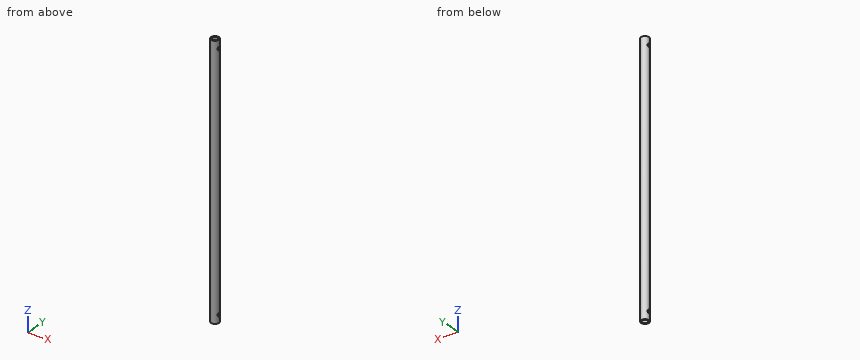
from build123d import *

# Parameters (mm, degrees)
ESQUISSE1_R                  = 3
ESQUISSE1_R_2                = 2
BOSS_EXTRU_1_DEPTH           = 199
ENL_V_MAT_EXTRU_1_DEPTH      = 200.045220993
ENL_V_MAT_EXTRU_1_DEPTH_BACK = 200.045220993
ESQUISSE2_R                  = 1.25


with BuildPart() as part:
    # Esquisse1 → Boss.-Extru.1 (new body)
    with BuildSketch(Plane.XY):
        Circle(ESQUISSE1_R)
        Circle(ESQUISSE1_R_2, mode=Mode.SUBTRACT)
    extrude(amount=BOSS_EXTRU_1_DEPTH)

    # Esquisse2 → Enlèv. mat.-Extru.1 (cut, two sides: drawn at the far end of the back side and taken through both)
    with BuildSketch(Plane(origin=(0, 0, 0), x_dir=(0, 0, -1), z_dir=(1, 0, 0)).offset(-ENL_V_MAT_EXTRU_1_DEPTH_BACK)):
        with Locations((-6, 0)):
            Circle(ESQUISSE2_R)
        with Locations((-193, 0)):
            Circle(ESQUISSE2_R)
    extrude(amount=ENL_V_MAT_EXTRU_1_DEPTH + ENL_V_MAT_EXTRU_1_DEPTH_BACK, mode=Mode.SUBTRACT)


solid = part.part
Input: part model. Units: mm. Frame: model coordinates. Give positions to 0.01 mm unless a question says otherwise; leave off trailing zeros. Loops run counter-clockwise (first coordinate to the right, second up) from the corner with the lowest first, then second, coordinate; pieces in that order, holes last. Notation, with made-up numbers: (32, 4.5) -> (76, 4.5) arc R19 ccw to (76, 36.5) -> close; hole circle Ø6 at (42.5, 17.5). An arc over 180 degrees is marked (long way). Answer as a JSON object with one key per item and string values. Group by question number.
Item 1: Cut plane A-A, the plane x = 0. Return the cut outline in (y, z).
Item 2: Pin query (flat end, axial travel): P1, Ø1, axis at x = -1, z = 147.5, coming from the +Y side; P2, Ø1.5, axis at y = -1, z = 28.5, coming from the +X side; P3, Ø1, axis at y = 2, z = 20, coming from the -X side. Return the tip coordinate at first contact, or that it passes through.
Item 3: Line query: probe 1 along Z at (x, y) = (2.15, 0); probe 2 along X at (y, z) = (0.25, 111); probe 3 along Y at (x, z) = (0, 12). Output: solid intervals per line, ascending.
Item 4: Cut plane B-B, the plane z = 30. Return the cut outline in (x, y), and give its area (3 significant figures).
Checks:
{
 "1": {"outline": "(-3, 0) -> (-2, 0) -> (-2, 199) -> (-3, 199) -> close; (2, 0) -> (3, 0) -> (3, 199) -> (2, 199) -> close"},
 "2": {"P1": "stops at y = 2.96", "P2": "stops at x = 2.99", "P3": "stops at x = -2.6"},
 "3": {"probe 1": "z = 0 to 4.75, 7.25 to 191.75, 194.25 to 199", "probe 2": "x = -2.99 to -1.98, 1.98 to 2.99", "probe 3": "y = -3 to -2, 2 to 3"},
 "4": {"outline": "circle Ø6 at (0, 0); hole circle Ø4 at (0, 0)", "area": "15.7 mm²"}
}
